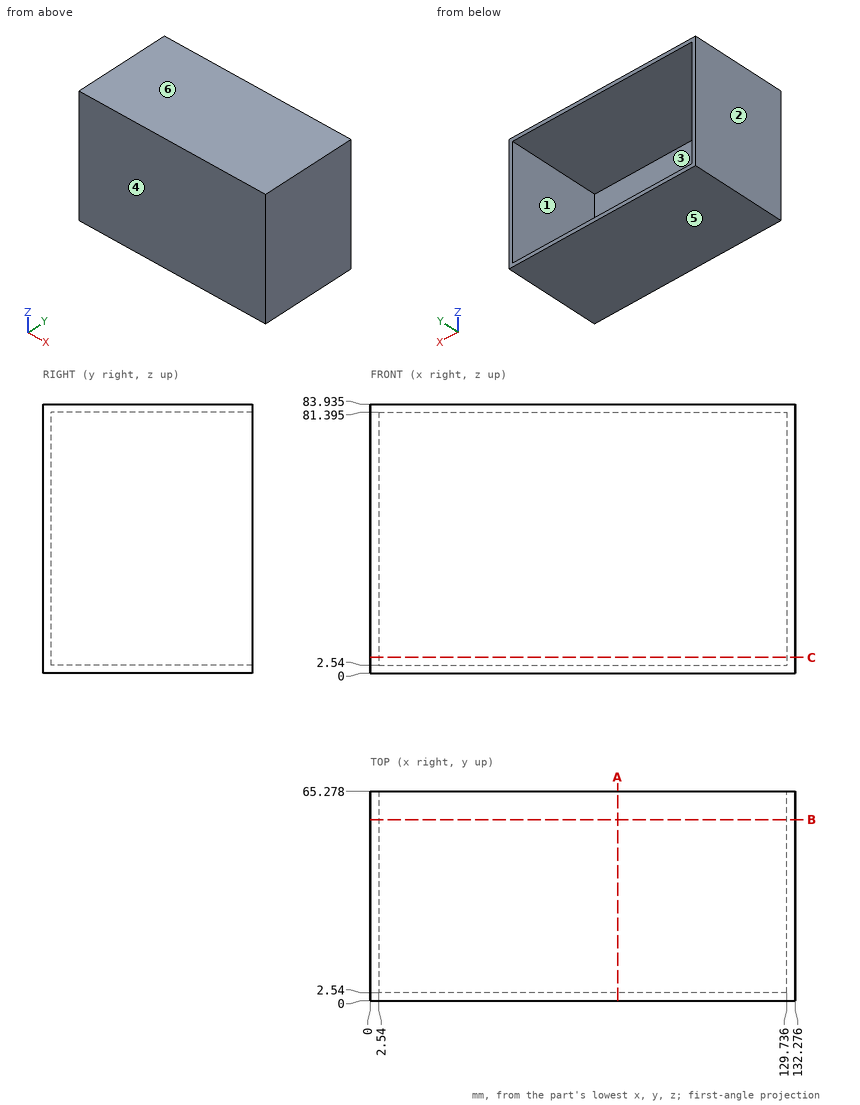
Drawing for the job (mm, zero at the part's lowest x, y, z). A direction names the side the tool comes from. Round coordinates to 2 decimals unless told otherwise and drop trailing zeros. Order: outer loops, then holes, each group sorted by start corner. A loop starts at its lowest first (then second) coordinate and runs counter-clockwise, first axis right, second up.
Item 1: Saw through at B-B on y = 56.5. Write the cut outline in (x, z) (1 decimal).
Item 2: Tool access for the marked faces 1 and 2: list every direction of +Z, -Z, +X, -X, +Y, -Y with a clear straight run to the whole face (end or side of a thin tool).
Item 3: Mould opens along Z. For the marked faces 3, 4, 5 and 6 say: pulls with the +Z half, pulls with the -Z half, needs draft (parallel to the pull), parting line crosses it, or undercut.
Item 4: Saw through at C-C on z = 5. Write the cut outline in (x, y) (1 decimal).
Item 5: Saw through at A-A on x = 77. Write the cut outline in (y, z) (1 decimal).
Item 6: Probe line 1 along X through (y, z) = (33.5, 22) (1 decimal); line 2 along Z through (x, y) = (103.5, 5) (1 decimal); line 3 along Y through (x, z) = (120, 26). List the from-to ranges inside material, lowest first.
Reported:
1. outline: (0, 0) - (132.3, 0) - (132.3, 83.9) - (0, 83.9) - close; hole (2.5, 2.5) - (129.7, 2.5) - (129.7, 81.4) - (2.5, 81.4) - close
2. face 1: +Y
2. face 2: +Z, -Z, -X, +Y, -Y
3. face 3: undercut
3. face 4: needs draft
3. face 5: pulls with the -Z half
3. face 6: pulls with the +Z half
4. outline: (0, 0) - (132.3, 0) - (132.3, 65.3) - (129.7, 65.3) - (129.7, 2.5) - (2.5, 2.5) - (2.5, 65.3) - (0, 65.3) - close
5. outline: (0, 0) - (65.3, 0) - (65.3, 2.5) - (2.5, 2.5) - (2.5, 81.4) - (65.3, 81.4) - (65.3, 83.9) - (0, 83.9) - close
6. line 1: x = 0 to 2.5, 129.7 to 132.3
6. line 2: z = 0 to 2.5, 81.4 to 83.9
6. line 3: y = 0 to 2.54
